from build123d import *

# Parameters (mm, degrees)
CROQUIS2_R       = 2
PAREDMOVIL_DEPTH = 110
VISAGRA_REACH    = 130.083
CROQUIS3_W       = 12
CROQUIS3_H       = 16
CROQUIS3_W_2     = 56


with BuildPart() as part:
    # Croquis2 → ParedMovil (new body)
    with BuildSketch(Plane.XY):
        with BuildLine():
            Line((27.5, 0), (32.5, 0))
            ThreePointArc((32.5, 0), (-1.757573948, -32.452441107), (-32.309903619, 3.510004003))
            Line((-32.309903619, 3.510004003), (-24.5, 3.510004003))
            Line((-24.5, 3.510004003), (-24.5, -12.489995997))
            ThreePointArc((-24.5, -12.489995997), (6.422616289, -26.739483914), (27.5, 0))
        make_face()
        with Locations((-28.5, 0)):
            Circle(CROQUIS2_R, mode=Mode.SUBTRACT)
    extrude(amount=PAREDMOVIL_DEPTH)

    # Croquis3 → Visagra (cut, up to next)
    with BuildSketch(Plane(origin=(-24.5, 0, 0), x_dir=(0, 0, -1), z_dir=(1, 0, 0)), mode=Mode.PRIVATE) as visagra_sk1:
        with Locations((-104, -4.489995997)):
            Rectangle(CROQUIS3_W, CROQUIS3_H)
    visagra_tool1 = extrude(visagra_sk1.sketch, amount=-VISAGRA_REACH, mode=Mode.PRIVATE) & part.part
    # Croquis3 → Visagra (cut, up to next)
    with BuildSketch(Plane(origin=(-24.5, 0, 0), x_dir=(0, 0, -1), z_dir=(1, 0, 0)), mode=Mode.PRIVATE) as visagra_sk2:
        with Locations((-6, -4.489995997)):
            Rectangle(CROQUIS3_W, CROQUIS3_H)
    visagra_tool2 = extrude(visagra_sk2.sketch, amount=-VISAGRA_REACH, mode=Mode.PRIVATE) & part.part
    # Croquis3 → Visagra (cut, up to next)
    with BuildSketch(Plane(origin=(-24.5, 0, 0), x_dir=(0, 0, -1), z_dir=(1, 0, 0)), mode=Mode.PRIVATE) as visagra_sk3:
        with Locations((-55, -4.489995997)):
            Rectangle(CROQUIS3_W_2, CROQUIS3_H)
    visagra_tool3 = extrude(visagra_sk3.sketch, amount=-VISAGRA_REACH, mode=Mode.PRIVATE) & part.part
    add(visagra_tool1.solids().sort_by_distance((-24.5, -4.489996, 104))[0], mode=Mode.SUBTRACT)
    add(visagra_tool2.solids().sort_by_distance((-24.5, -4.489996, 6))[0], mode=Mode.SUBTRACT)
    add(visagra_tool3.solids().sort_by_distance((-24.5, -4.489996, 55))[0], mode=Mode.SUBTRACT)


solid = part.part
Model file for the job. Use its own axes, mm. A direction names the side the tool comes from. Give positions to 0.01 mm unless a question says otherwise; leave off trailing zeros. Loops run counter-clockwise (first coordinate to the right, second up) from the corner with the lowest first, then second, coordinate; pieces in that order, holes last. Notation, with made-up numbers: (89.5, 79.25) - (111.5, 79.25) arc R16 cw to (111.5, 92.25) - close; hole circle Ø6 at (80.25, -13). An arc over 180 degrees is marked (long way). Use one line per item in the form item = value.
(1) Cut at C-C (y = -9). Give the cut face in (x, z).
Determined:
outline = (-31.23, 12) - (-24.5, 12) - (-24.5, 27) - (-31.23, 27) - close; (-31.23, 83) - (-24.5, 83) - (-24.5, 98) - (-31.23, 98) - close; (25.99, 0) - (31.23, 0) - (31.23, 110) - (25.99, 110) - close
(2) Pull direction Z, two halves, no side cores. Call faces 1 (the face through (-28, -5, 83)), 2 (the face through (4, -28, 0)), 3 (the face through (4, -28, 110)), 4 (the face through (-27, -12.49, 6)): pulls with the +Z half, pulls with the -Z half, needs draft (parallel to the pull), parting line crosses it, or undercut.
Determined:
face_1 = undercut
face_2 = pulls with the -Z half
face_3 = pulls with the +Z half
face_4 = needs draft
(3) Cut at D-D (x = 0). Give the cut face in (y, z), then the cut area to 3 significant figures.
Determined:
outline = (-32.5, 0) - (-27.5, 0) - (-27.5, 110) - (-32.5, 110) - close
area = 550 mm^2
(4) Drop flat-ended pins along their axis: P1, Ø10, axis at y = -23, z = 77, coming from the +X side; P2, Ø6.5, axis at x = -26.5, y = -4, coming from the +Z side; P3, Ø5.5, axis at x = 30, z = 30.5, coming from the +Y side. Give the stop position or say it passes through.
Determined:
P1 = 27.06
P2 = 98
P3 = 0
(5) Cut at A-A (y = -23.5). Give the cut face in (x, z), then the cut area to 3 significant figures.
Determined:
outline = (-22.45, 0) - (-14.28, 0) - (-14.28, 110) - (-22.45, 110) - close; (14.28, 0) - (22.45, 0) - (22.45, 110) - (14.28, 110) - close
area = 1,800 mm^2
(6) Drill centre lines: L1, parallel to Y at x = -28.5, z = 20; L2, parallel to X at y = -17, z = 34.5; L3, parallel to X at y = -17.5, z = 37. Where is each one in solid material? Low to high.
Determined:
L1 = -15.62 to -2, 2 to 3.51
L2 = -27.7 to -21.62, 21.62 to 27.7
L3 = -27.39 to -21.21, 21.21 to 27.39
(7) 3-axis set-ups, long thin cutter, end or side, ignore diameter. For faces 5 (the face through (30, 0, 54)), 6 (the face through (-28, -5, 12)), 7 (the face through (-28, -5, 98)), 8 (the face through (-27, -12.49, 55)): which of +Z, -Z, +X, -X, +Y, -Y reach the whole face in a straight line?
Determined:
face_5 = +Z, -Z, +X, +Y
face_6 = -Z, -X, +Y
face_7 = +Z, -X, +Y
face_8 = -X, +Y
(8) Cut at B-B (x = -28.5). Give the cut face in (y, z).
Determined:
outline = (-15.62, 0) - (-12.49, 0) - (-12.49, 12) - (-2, 12) - (-2, 27) - (-12.49, 27) - (-12.49, 83) - (-2, 83) - (-2, 98) - (-12.49, 98) - (-12.49, 110) - (-15.62, 110) - close; (2, 12) - (3.51, 12) - (3.51, 27) - (2, 27) - close; (2, 83) - (3.51, 83) - (3.51, 98) - (2, 98) - close
